Autodesk Inventor part; units mm, degrees
ref_plane "YZ Plane" through (0, 0, 0) normal (1, 0, 0) x (0, 1, 0)
ref_plane "XZ Plane" through (0, 0, 0) normal (0, 1, 0) x (-1, 0, 0)
ref_plane "XY Plane" through (0, 0, 0) normal (0, 0, 1) x (1, 0, 0)
sketch "Sketch1" plane through (0, 0, 0) normal (0, 0, 1) x (1, 0, 0)
  line L0 (-3.981, 7.2547) -> (33.019, 7.2547)
  line L1 (33.019, 7.2547) -> (36.269, -7.7453)
  line L2 (-7.231, -7.7453) -> (-3.981, 7.2547)
  line L3 (-0.731, -1.2453) -> (29.769, -1.2453)
  line L4 (29.769, -1.2453) -> (29.769, -7.7453)
  line L5 (-0.731, -1.2453) -> (-0.731, -7.7453)
  line L6 (36.269, -7.7453) -> (29.769, -7.7453)
  line L7 (-0.731, -7.7453) -> (-7.231, -7.7453)
  point P0 (0, 0)
  dimension "d0" = 37
  dimension "d1" = 43.5
  dimension "d4" = 30.5
extrude "Extrusion1" add sketch "Sketch1" along normal blind 300
sketch "Sketch2" plane through (-3.981, 7.2547, 0) normal (0, 1, 0) x (1, 0, 0)
  line L0 (37, -300) -> (0, -300)
  line L1 (0, 0) -> (37, 0)
  point P0 (3.981, 0)
  point P1 (18.5, -10)
  point P2 (18.5, -132)
  point P3 (18.5, -168)
  point P4 (18.5, -290)
  dimension "d9" = 10
  dimension "d10" = 10
  dimension "d11" = 36
hole "Hole1" at (14.519, 7.2547, 10) at (14.519, 7.2547, 132) at (14.519, 7.2547, 168) at (14.519, 7.2547, 290) direction (0, -1, 0) diameter 4.978 end through all
chamfer "Chamfer1" distance 0.3 angle 45 4 edges at (14.519, 7.2547, 287.511) (14.519, 7.2547, 7.511) (14.519, -1.2453, 129.511) (14.519, -1.2453, 165.511)
properties part number "szyna" material "Stainless Steel"
CAD build for the part. Positions are in the model's coordinates, mm. A direction names the side the tool comes from. Give positions to 0.01 mm unless a question says otherwise; leave off trailing zeros. Write each loop counter-clockwise with the first axis right and the second up, starting at its lowest first coordinate (ties: lowest second). Pieces come first, ordered by that corner, then holes. Notation, with made-up numbers: M -17.5,22 L -6.5,22 A23 ccw -6.5,40 Z; hole C 3,85 d7. An arc over 180 degrees is marked long. Put each result on its own line as item: value. Start each with the question number.
(1) Flat gauge pins, fed straight in: pin 1 Ø8 at (x, z) = (14.519, 10) entering from -Y; pin 2 Ø1.5 at (y, z) = (-4, 169) entering from +X; pin 3 Ø3 at (y, z) = (-3.5, 151) entering from +X. Where does each tip first touch, or does it go through?
(2) Mould opens along Z. For faces 3 (the face through (14.41, 3.097, 129.513)), 4 (the face through (-4, -7.745, 148)), 5 (the face through (14, 2, 0)) say: +Z half, -Z half, draft (parallel to the pull), parting line (faces both ways), or undercut.
(3) Band-saw the part on C-C, the plane x = 24. Write the cut outline in (y, z), and give its area (3 significant figures).
(4) Probe L1, parallel to Z at x = 15, y = 1.5; L2, parallel to Z at x = 16, y = 6.5; L3, parallel to Y at x = 28.5, z = 186.5. List the from-to ranges inside material, lowest first.
(5) Which spindle directions (+Z, -Z, +X, -X, +Y, -Y) get a long thin tool onto all of the face, cutting with end or side? Do faces 1 (the face through (-5.63, -0.35, 147.9)), 2 (the face through (-0.731, -4, 148)). Say none if no direction does.
(6) Band-saw the part on B-B, the plane y = 2.5. Write the cut outline in (x, z), and give its area (3 significant figures).
(7) Band-saw the part on A-A, the plane z = 132. Write the cut outline in (x, y), and give its area (3 significant figures).
Response values:
1. pin 1: stops at y = -1.25
1. pin 2: stops at x = 35.62
1. pin 3: stops at x = 35.67
2. face 3: undercut
2. face 4: draft
2. face 5: -Z half
3. outline: M -1.25,0 L 7.25,0 L 7.25,300 L -1.25,300 Z
3. area: 2,550 mm2
4. L1: z = 0 to 7.56, 12.44 to 129.56, 134.44 to 165.56, 170.44 to 287.56, 292.44 to 300
4. L2: z = 0 to 8, 12 to 130, 134 to 166, 170 to 288, 292 to 300
4. L3: y = -1.25 to 7.25
5. face 1: +Z, -Z, -X, +Y
5. face 2: +Z, -Z, -Y
6. outline: M -5.01,0 L 34.05,0 L 34.05,300 L -5.01,300 Z; hole C 14.52,10 d4.98; hole C 14.52,132 d4.98; hole C 14.52,168 d4.98; hole C 14.52,290 d4.98
6. area: 11,600 mm2
7. outline: M -7.23,-7.75 L -0.73,-7.75 L -0.73,-1.25 L 11.73,-1.25 L 12.03,-0.95 L 12.03,7.25 L -3.98,7.25 Z; M 17.01,-0.95 L 17.31,-1.25 L 29.77,-1.25 L 29.77,-7.75 L 36.27,-7.75 L 33.02,7.25 L 17.01,7.25 Z
7. area: 363 mm2
